Verification items for this drawing (mm, ordinates from the low corner). Coordinates: 2 decimals unless noted, no trailing zeros. Loops run counter-clockwise (first coordinate to the right, second up) from the corner with the lowest first, then second, coordinate; pieces in that order, holes last. Notation, with made-up numbers: (56.5, 48) - (89.5, 48) arc R24 cw to (89.5, 68) - close; hole circle Ø5 at (-18, 61). An arc over 180 degrees is marked (long way). One line per item, written item: value. Start each with the question number.
(1) Thickness scan on probe 1 along X at (y, z) = (2.15, 10); probe 2 along X at (y, z) = (1.7, 14.5); probe 3 along Z at (x, y) = (16, 2.4). Record the ranges inside material, lowest first. Write a range as [from, to].
(2) Section check C-C (y = 1.45). Record the boundary of the cut face in (x, z).
(3) Gauge pin test, flat ends, axial feed: P1, Ø2, axis at x = 26, z = 3, coming from the -Y side; P2, Ø1, axis at y = 4, z = 8.5, coming from the -X side; P3, Ø2, axis at y = 3.5, z = 25.5, coming from the +X side; P4, Ø1.5, axis at x = 9.5, y = 2.5, coming from the -Z side. Record the tip position at first contact, or that the pin passes through.
(4) Section check B-B (z = 15). Record the boundary of the cut face in (x, y).
(5) Section check D-D (y = 4.7). Record the boundary of the cut face in (x, z), plus the area to 3 significant figures.
(6) Section check A-A (x = 15). Record the boundary of the cut face in (y, z), plus the area to 3 significant figures.
(7) Draft check along X on the marked faces 1 and 2. Enter one of: +X half, -X half, draft (parallel to the pull), parting line (faces both ways), or undercut.
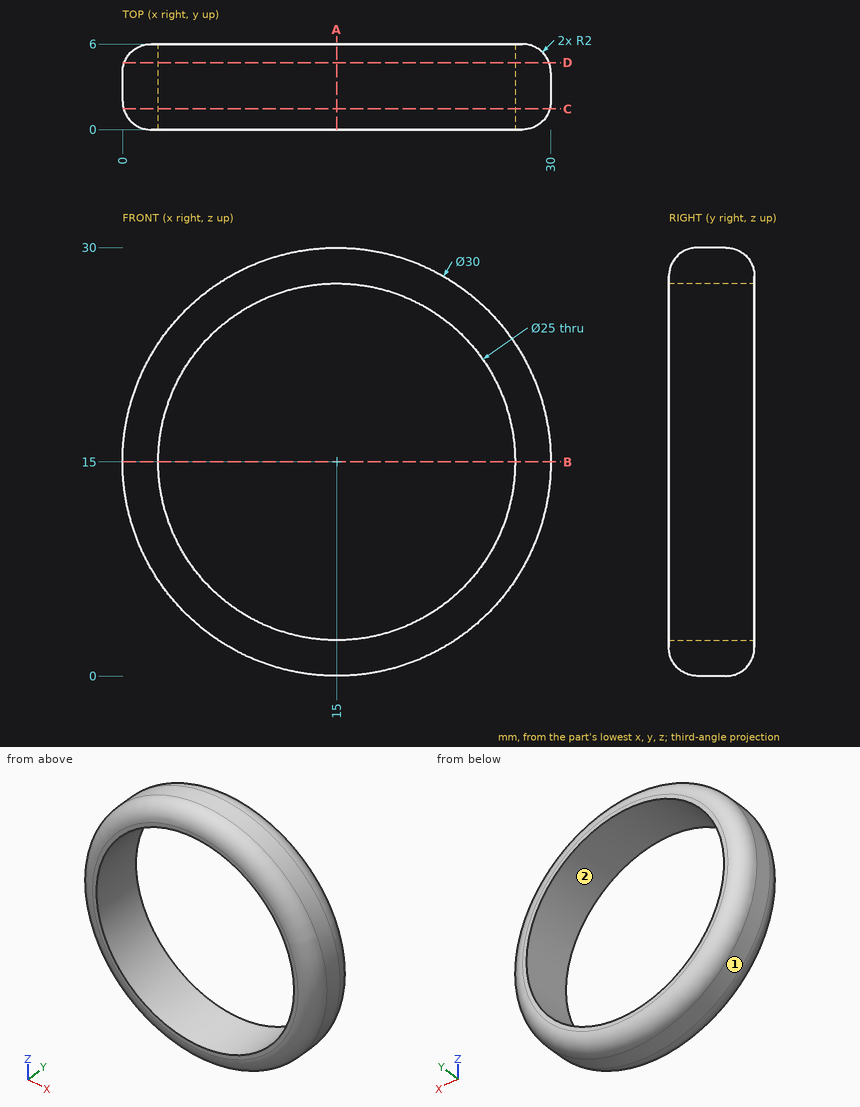
Responses:
1. probe 1: x = [0.86, 3.54], [26.46, 29.14]
1. probe 2: x = [0.03, 2.51], [27.49, 29.97]
1. probe 3: z = [0.03, 2.54], [27.46, 29.97]
2. outline: circle Ø29.85 at (15, 15); hole circle Ø25 at (15, 15)
3. P1: passes through
3. P2: stops at x = 1.25
3. P3: stops at x = 26.61
3. P4: stops at z = 0.77
4. outline: (0, 2) arc R2 ccw to (2, 0) - (2.5, 0) - (2.5, 6) - (2, 6) arc R2 ccw to (0, 4) - close; (27.5, 0) - (28, 0) arc R2 ccw to (30, 2) - (30, 4) arc R2 ccw to (28, 6) - (27.5, 6) - close
5. outline: circle Ø29.75 at (15, 15); hole circle Ø25 at (15, 15)
5. area: 204 mm²
6. outline: (0, 2) arc R2 ccw to (2, 0) - (4, 0) arc R2 ccw to (6, 2) - (6, 2.5) - (0, 2.5) - close; (0, 27.5) - (6, 27.5) - (6, 28) arc R2 ccw to (4, 30) - (2, 30) arc R2 ccw to (0, 28) - close
6. area: 26.6 mm²
7. face 1: parting line
7. face 2: undercut
